```python
from build123d import *

# Parameters (mm, degrees)
SKETCH1_W                          = 69.85
SKETCH1_H                          = 47.625
BOSS_EXTRUDE1_DEPTH                = 19.05
CUT_EXTRUDE1_REACH                 = 21.05
SKETCH2_W                          = 50.8
SKETCH2_H                          = 28.575
F_5_16_24_TAPPED_HOLE1_D           = 6.9088
F_5_16_24_TAPPED_HOLE1_DEPTH       = 19.06
F_5_16_24_TAPPED_HOLE1_CSINK_D     = 9.2075
F_5_16_24_TAPPED_HOLE1_CSINK_ANGLE = 90
F_5_16_24_TAPPED_HOLE1_TIP         = 2.075612922
F_5_16_CLEARANCE_HOLE1_D           = 8.2042
F_5_16_CLEARANCE_HOLE1_CSINK_D     = 9.4742
F_5_16_CLEARANCE_HOLE1_CSINK_ANGLE = 90
CHAMFER1_SIZE                      = 1.5


with BuildPart() as part:
    # Sketch1 → Boss-Extrude1 (new body)
    with BuildSketch(Plane(origin=(0, 0, 0), x_dir=(1, 0, 0), z_dir=(0, 1, 0))):
        Rectangle(SKETCH1_W, SKETCH1_H)
    extrude(amount=BOSS_EXTRUDE1_DEPTH)

    # Sketch2 → Cut-Extrude1 (cut, up to next)
    with BuildSketch(Plane(origin=(0, 19.05, 0), x_dir=(1, 0, 0), z_dir=(0, 1, 0)), mode=Mode.PRIVATE) as cut_extrude1_sk1:
        with Locations((9.525, 9.525)):
            Rectangle(SKETCH2_W, SKETCH2_H)
    cut_extrude1_tool1 = extrude(cut_extrude1_sk1.sketch, amount=-CUT_EXTRUDE1_REACH, mode=Mode.PRIVATE) & part.part
    add(cut_extrude1_tool1.solids().sort_by_distance((9.525, 19.05, -9.525))[0], mode=Mode.SUBTRACT)

    # 5/16-24 Tapped Hole1
    with Locations(Plane.ZY.offset(34.925)):
        with Locations((-14.2875, 9.525), (11.1125, 9.525)):
            CounterSinkHole(F_5_16_24_TAPPED_HOLE1_D / 2, F_5_16_24_TAPPED_HOLE1_CSINK_D / 2, depth=F_5_16_24_TAPPED_HOLE1_DEPTH, counter_sink_angle=F_5_16_24_TAPPED_HOLE1_CSINK_ANGLE)
            with Locations((0, 0, -(F_5_16_24_TAPPED_HOLE1_DEPTH + F_5_16_24_TAPPED_HOLE1_TIP / 2))):  # 118° drill point
                Cone(0, F_5_16_24_TAPPED_HOLE1_D / 2, F_5_16_24_TAPPED_HOLE1_TIP, mode=Mode.SUBTRACT)

    # 5/16 Clearance Hole1 (through all)
    with Locations(Plane(origin=(0, 0, 4.7625), x_dir=(-1, 0, 0), z_dir=(0, 0, -1))):
        with Locations((3.175, 9.525), (-22.225, 9.525)):
            CounterSinkHole(F_5_16_CLEARANCE_HOLE1_D / 2, F_5_16_CLEARANCE_HOLE1_CSINK_D / 2, counter_sink_angle=F_5_16_CLEARANCE_HOLE1_CSINK_ANGLE)

    # Chamfer1
    chamfer1_edges = [part.edges().sort_by_distance(p)[0] for p in [
        (-25.4, 0, -23.8125),
        (-25.4, 19.05, -23.8125),
        (9.525, 0, 4.7625),
        (34.925, 9.525, 4.7625),
        (-15.875, 9.525, -23.8125),
        (9.525, 19.05, 4.7625),
    ]]
    chamfer(chamfer1_edges, length=CHAMFER1_SIZE)


solid = part.part
```
Model file for the job. Use its own axes, mm. A direction names the side the tool comes from. Coordinates: 2 decimals unless noted, no trailing zeros. Order: outer loops, then holes, each group sorted by start corner. A loop starts at its lowest first (then second) coordinate and runs counter-clockwise, first axis right, second up. Notation, with made-up numbers: (-25.5, -29.5) -> (-7.5, -29.5) arc R20 cw to (-7.5, -24.5) -> close; hole circle Ø6 at (-18.75, 0.5). An arc over 180 degrees is marked (long way). Answer as a JSON object with one key per item and string values. Group by question number.
1) Cut at D-D, the plane z = 19.5. Write the cut outline in (x, y) (3 decimals).
2) Flat gauge pins, fed straight in: pin 1 (9 mm diameter, centred on y = 9.52, z = -14.29, fed in from -X); pin 2 (5.5 mm diameter, centred on y = 11, z = -10, fed in from +X) (3 decimals). Where does each tip first touch, or does it go through?
3) Cut at A-A, the plane x = 28. Write the cut outline in (y, z), then the cut area to 3 significant figures.
4) Which spindle directions (+Z, -Z, +X, -X, +Y, -Y) get a long thin tool onto all of the face, cutting with end or side? Do faces 1 (the face through (9.88, 0.74, 5.52)), 2 (the face through (-24.69, 11.86, 13.66)), 3 (the face through (8, 10, 4.762)). Say none if no direction does.
5) Cut at B-B, the plane y = 2.5. Write the cut outline in (x, z) (1 decimal).
6) Drill centre lines: L1, parallel to Z at x = -19, y = 11.25; L2, parallel to Z at x = -16.5, y = 9.75; L3, parallel to X at y = 5.5, z = -1 (3 decimals). Where is each one in solid material? Low to high.
7) Pull direction Z, two halves, no side cores. Call faces 4 (the face through (0, 14, 23.812)), 5 (the face through (-24.7, 10.563, -17.582)), 6 (the face through (-26, 9, -23.812)): +Z half, -Z half, draft (parallel to the pull), parting line (faces both ways), or undercut.
Check values:
{
 "1": {"outline": "(-34.925, 0) -> (34.925, 0) -> (34.925, 19.05) -> (-34.925, 19.05) -> close; hole circle Ø8.204 at (-3.175, 9.525); hole circle Ø8.204 at (22.225, 9.525)"},
 "2": {"pin 1": "stops at x = -34.83", "pin 2": "stops at x = -15.875"},
 "3": {"outline": "(0, 6.26) -> (1.5, 4.76) -> (17.55, 4.76) -> (19.05, 6.26) -> (19.05, 23.81) -> (0, 23.81) -> close", "area": "361 mm²"},
 "4": {"face 1": "-Z, +X, -Y", "face 2": "-X", "face 3": "-Z, +X, +Y, -Y"},
 "5": {"outline": "(-34.9, -23.8) -> (-17.4, -23.8) -> (-15.9, -22.3) -> (-15.9, 4.8) -> (33.4, 4.8) -> (34.9, 6.3) -> (34.9, 23.8) -> (-34.9, 23.8) -> close"},
 "6": {"L1": "z = -23.81 to -17.28, -11.29 to 8.12, 14.11 to 23.81", "L2": "z = -22.94 to -17.73, -10.84 to 7.67, 14.56 to 23.81", "L3": "x = -34.925 to -15.875"},
 "7": {"face 4": "+Z half", "face 5": "undercut", "face 6": "-Z half"}
}
